from build123d import *

# Parameters (mm, degrees)
F0_R     = 21.803991
F1_DEPTH = 12.5
F2_COUNT = 12
F3_DEPTH = 15


with BuildPart() as f1:
    # F0 (on Front) → F1 (new body)
    with BuildSketch(Plane.XZ):
        with BuildLine():
            ThreePointArc((-7.376443, 25.827786), (-16.176395, -21.443197), (26.8605, 0))
            ThreePointArc((26.8605, 0), (19.148304, 18.836903), (0.440374, 26.85689))
            ThreePointArc((0.440374, 26.85689), (-3.505999, 26.630705), (-7.376443, 25.827786))
        make_face()
        Circle(F0_R, mode=Mode.SUBTRACT)
        with BuildLine():
            ThreePointArc((-7.376443, 25.827786), (-3.505999, 26.630705), (0.440374, 26.85689))
            ThreePointArc((0.440374, 26.85689), (0.403553, 28.129504), (0, 29.337))
            ThreePointArc((0, 29.337), (-0.67184, 30.552787), (-1.42822, 31.717861))
            ThreePointArc((-1.42822, 31.717861), (-4.121867, 31.308688), (-6.829632, 31.006751))
            ThreePointArc((-6.829632, 31.006751), (-7.258695, 29.685611), (-7.592974, 28.337366))
            ThreePointArc((-7.592974, 28.337366), (-7.670253, 27.066567), (-7.376443, 25.827786))
        make_face()
    extrude(amount=F1_DEPTH)



with BuildPart() as f2_1:
    # F2: instance of F1
    add(f1.part.rotate(Axis((0, 0, 0), (0, 1, 0)), 1 * 360 / F2_COUNT))


with BuildPart() as f2_2:
    # F2: instance of F1
    add(f1.part.rotate(Axis((0, 0, 0), (0, 1, 0)), 2 * 360 / F2_COUNT))


with BuildPart() as f2_3:
    # F2: instance of F1
    add(f1.part.rotate(Axis((0, 0, 0), (0, 1, 0)), 3 * 360 / F2_COUNT))


with BuildPart() as f2_4:
    # F2: instance of F1
    add(f1.part.rotate(Axis((0, 0, 0), (0, 1, 0)), 4 * 360 / F2_COUNT))


with BuildPart() as f2_5:
    # F2: instance of F1
    add(f1.part.rotate(Axis((0, 0, 0), (0, 1, 0)), 5 * 360 / F2_COUNT))


with BuildPart() as f2_6:
    # F2: instance of F1
    add(f1.part.rotate(Axis((0, 0, 0), (0, 1, 0)), 6 * 360 / F2_COUNT))


with BuildPart() as f2_7:
    # F2: instance of F1
    add(f1.part.rotate(Axis((0, 0, 0), (0, 1, 0)), 7 * 360 / F2_COUNT))


with BuildPart() as f2_8:
    # F2: instance of F1
    add(f1.part.rotate(Axis((0, 0, 0), (0, 1, 0)), 8 * 360 / F2_COUNT))


with BuildPart() as f2_9:
    # F2: instance of F1
    add(f1.part.rotate(Axis((0, 0, 0), (0, 1, 0)), 9 * 360 / F2_COUNT))


with BuildPart() as f2_10:
    # F2: instance of F1
    add(f1.part.rotate(Axis((0, 0, 0), (0, 1, 0)), 10 * 360 / F2_COUNT))


with BuildPart() as f2_11:
    # F2: instance of F1
    add(f1.part.rotate(Axis((0, 0, 0), (0, 1, 0)), 11 * 360 / F2_COUNT))


with BuildPart() as f1_1:
    add(f1.part)

    add(f2_1.part)  # F3 merges F2_1

    add(f2_2.part)  # F3 merges F2_2

    add(f2_3.part)  # F3 merges F2_3

    add(f2_4.part)  # F3 merges F2_4

    add(f2_5.part)  # F3 merges F2_5

    add(f2_6.part)  # F3 merges F2_6

    add(f2_7.part)  # F3 merges F2_7

    add(f2_8.part)  # F3 merges F2_8

    add(f2_9.part)  # F3 merges F2_9

    add(f2_10.part)  # F3 merges F2_10

    add(f2_11.part)  # F3 merges F2_11
    # F0 (on Front) → F3 (join)
    with BuildSketch(Plane.XZ):
        Circle(F0_R)
        with BuildLine():
            ThreePointArc((5.071371, 0), (3.55472, -3.61701), (-0.088088, -5.070606))
            ThreePointArc((-0.088088, -5.070606), (-3.767643, -3.394653), (-5.052327, 0.439082))
            ThreePointArc((-5.052327, 0.439082), (-2.054693, 4.63649), (3.068356, 4.03782))
            ThreePointArc((3.068356, 4.03782), (4.543103, 2.253667), (5.071371, 0))
        make_face(mode=Mode.SUBTRACT)
    extrude(amount=F3_DEPTH)


solid = f1_1.part
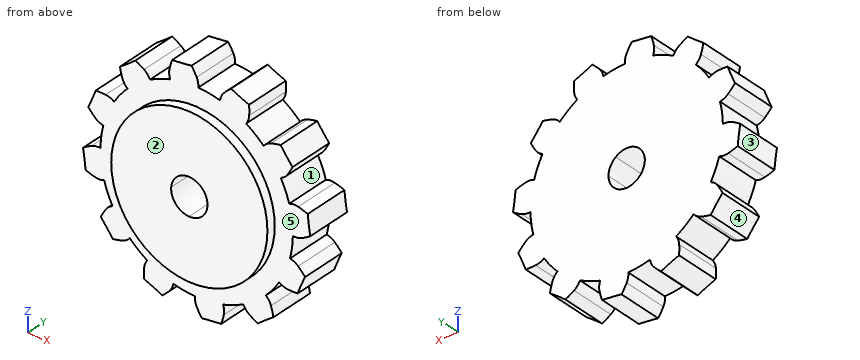
Build history of the part. All positions in model axes, mm. Face numbers are marked on the shaded views. A direction names the side the tool comes from. Give positions to 0.01 mm unless a question says otherwise; leave off trailing zeros. Order: outer loops, then holes, each group sorted by start corner. A loop starts at its lowest first (then second) coordinate and runs counter-clockwise, first axis right, second up. Notation, with made-up numbers: M 45.5,69 L 79.5,69 A26 cw 79.5,87 Z; hole C -22,-5 d8. An arc over 180 degrees is marked long. Put each result on its own line as item: value.
Item 1: Slice it at A-A, the plane z = 11.5. Write the cut outline in (x, y).
From the geometry:
outline: M -29.42,-12.5 L -18.52,-12.5 L -18.52,-15 L 18.52,-15 L 18.52,-12.5 L 24.27,-12.5 L 24.27,0 L -29.42,0 Z
Item 2: Probe line 1 (Y direction, x = 21.5, z = -16); line 2 (Z direction, x = -24.5, y = -3.25); line 3 (X direction, y = -6.5, z = 3.5). List the from-to ranges inside material, lowest first. Write a range as [from, to].
From the geometry:
line 1: y = [-12.5, 0]
line 2: z = [-19.95, -13.66], [-11.01, 14.52]
line 3: x = [-26.63, -3.67], [3.67, 31.39]
Item 3: Two-plate mould, pull along Z, no slides. Class the marked faces 1, 2 and 3: +Z half, -Z half, draft (parallel to the pull), parting line (faces both ways), or undercut.
From the geometry:
face 1: undercut
face 2: draft
face 3: -Z half
Item 4: Flat gauge pins, fed straight in: pin 1 Ø8 at (x, y) = (18, -6.5) entering from -Z; pin 2 Ø2 at (x, y) = (-25, -8.5) entering from -Z; pin 3 Ø3 at (x, y) = (-22.5, -8.5) entering from +Z. Where does each tip first touch, or does it go through?
From the geometry:
pin 1: stops at z = -26.75
pin 2: stops at z = -20.63
pin 3: stops at z = 23.74
Item 5: Slice it at B-B, the plane x = -15.5. Write the cut outline in (y, z), plus the area to 3 significant figures.
From the geometry:
outline: M -15,-15.34 L -12.5,-15.34 L -12.5,-21.94 L 0,-21.94 L 0,25.92 L -12.5,25.92 L -12.5,15.34 L -15,15.34 Z
area: 675 mm2
Item 6: 3-axis set-ups, long thin cutter, end or side, ignore diameter. For the marked faces 4 and 5: which of +Z, -Z, +X, -X, +Y, -Y reach the whole face in a straight line?
From the geometry:
face 4: -Z, -X, +Y, -Y
face 5: -Y
